The listing builds one solid part. Answer for the finished solid, in the listing's coordinates (mm). A direction names the side the tool comes from. Coordinates: 2 decimals unless noted, no trailing zeros. Loops run counter-clockwise (first coordinate to the right, second up) from the corner with the lowest first, then second, coordinate; pieces in that order, holes last. Notation, with made-up numbers: M 34,38.5 L 70,38.5 A20 ccw 70,50.5 Z; hole C 59.25,0 d9. An arc over 180 degrees is marked long. Return JSON: item names as keys, results as strings. Group by question number.
1. Given P1, Ø1.5, axis at x = 13.5, z = 8, coming from the -Y side; P2, Ø1.5, axis at x = -7, z = 6.5, coming from the +Y side; P3, Ø3, axis at x = -9.5, z = 3, coming from the -Y side, each flat-ended and moving along its own axis, determine where each tip first touches the part or whether it passes through.
2. Section D-D (x = 5) is taken. Write down the section's boundary in (y, z) (3 decimals).
3. Section C-C (y = -15) is taken. Write down the section's boundary in (x, z).
4. Straight lines are drawn through the part: L1, parallel to X at y = 10, z = 2.75; L2, parallel to Z at x = 6.5, y = -7.5; L3, parallel to X at y = 16.5, z = 11.25. For each, find the intervals that lie inside material, in ascending order. Write a range as from..to.
5. Section A-A (z = 5.25) is taken. Write down the section's boundary in (x, y), then the cut area to 3 significant figures.
6. Which of the six approach directions +Z, -Z, +X, -X, +Y, -Y give full straight-line access (tool end or side, diameter ignored) to faces 1 (the face through (-1.73, -7.81, 20.96)), 2 (the face through (4.93, -18.68, 9.13))?
7. Section B-B (x = 1) is taken. Write down the section's boundary in (y, z).
```python
from build123d import *

# Parameters (mm, degrees)
SKETCH_1_R          = 8
EXTRUDE_1_DEPTH     = 24
SKETCH_2_R          = 42
EXTRUDE_2_DEPTH     = 18
SKETCH_3_OUTSIDE_W  = 110.238
SKETCH_3_OUTSIDE_H  = 110.238
CUT_EXTRUDE_1_DEPTH = 63.064482597


with BuildPart() as part:
    # 草图1 → 凸台-拉伸1 (new body)
    with BuildSketch(Plane.XY):
        Circle(SKETCH_1_R)
    extrude(amount=EXTRUDE_1_DEPTH)

    # 草图2 → 凸台-拉伸2 (add)
    with BuildSketch(Plane.XY):
        Circle(SKETCH_2_R)
    extrude(amount=EXTRUDE_2_DEPTH)

    # 草图3 outside → 切除-拉伸1 (cut, through all)
    with BuildSketch(Plane.XY.offset(18)):
        Rectangle(SKETCH_3_OUTSIDE_W, SKETCH_3_OUTSIDE_H)
        Polygon((20, 0), (17.320508076, 10), (10, 17.320508076), (0, 20), (-10, 17.320508076), (-17.320508076, 10), (-20, 0), (-17.320508076, -10), (-10, -17.320508076), (0, -20), (10, -17.320508076), (17.320508076, -10), align=None, mode=Mode.SUBTRACT)
    extrude(amount=-CUT_EXTRUDE_1_DEPTH, mode=Mode.SUBTRACT)


solid = part.part
```
Worked out:
{
 "1": {"P1": "y = -14.57", "P2": "y = 18.33", "P3": "y = -17.86"},
 "2": {"outline": "M -18.66,0 L 18.66,0 L 18.66,18 L 6.245,18 L 6.245,24 L -6.245,24 L -6.245,18 L -18.66,18 Z"},
 "3": {"outline": "M -12.32,0 L 12.32,0 L 12.32,18 L -12.32,18 Z"},
 "4": {"L1": "-17.32..17.32", "L2": "0..18", "L3": "-10.82..10.82"},
 "5": {"outline": "M -20,0 L -17.32,-10 L -10,-17.32 L 0,-20 L 10,-17.32 L 17.32,-10 L 20,0 L 17.32,10 L 10,17.32 L 0,20 L -10,17.32 L -17.32,10 Z", "area": "1,200 mm^2"},
 "6": {"face 1": "+Z", "face 2": "+Z, -Z, +X, -Y"},
 "7": {"outline": "M -19.73,0 L 19.73,0 L 19.73,18 L 7.94,18 L 7.94,24 L -7.94,24 L -7.94,18 L -19.73,18 Z"}
}
